Verification items for the finished model (mm, model axes). Face numbers are marked on the shaded views. Round coordinates to 2 decimals unless told otherwise and drop trailing zeros. Loops run counter-clockwise (first coordinate to the right, second up) from the corner with the lowest first, then second, coordinate; pieces in that order, holes last. Notation, with made-up numbers: M 68,-32.5 L 119,-32.5 A30 cw 119,5.5 Z; hole C -5.5,-2.75 d1. An arc over 180 degrees is marked long. One line per item, written item: value.
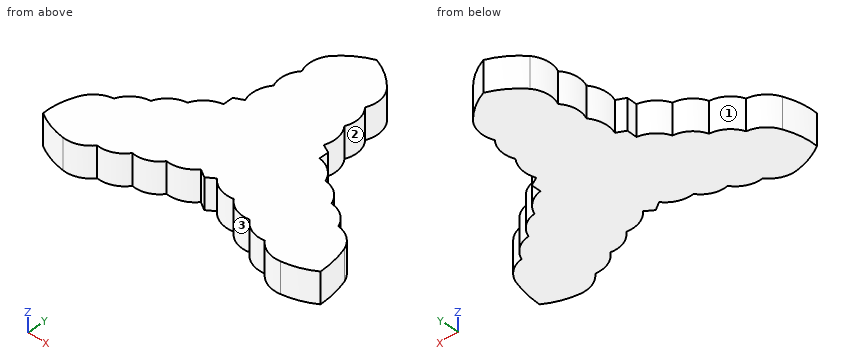
from build123d import *

# Parameters (mm, degrees)
F1_DEPTH = 7.9375


# Not quite as in the source:
# - a length typed as a fraction of an inch, garbled in the dataset ("3 / 203.2 mm" for 3/8 in), is restored


with BuildPart() as f1:
    # F0 (on Top) → F1 (new body)
    with BuildSketch(Plane.XY):
        with BuildLine():
            ThreePointArc((-0.0986067535, 34.0497419238), (-4.0682176485, 31.9659465467), (-7.4162920937, 28.9842672646))
            ThreePointArc((-7.4162920937, 28.9842672646), (-8.8119305122, 25.5953281623), (-8.2258973271, 21.977417171))
            ThreePointArc((-8.2258973271, 21.977417171), (-9.7181261566, 18.698842434), (-9.2097157612, 15.1327075437))
            ThreePointArc((-9.2097157612, 15.1327075437), (-10.6205392688, 11.8246856933), (-10.2093555033, 8.2519613206))
            Line((-10.2093555033, 8.2519613206), (-12.369341217, 7.1464567445))
            Line((-12.369341217, 7.1464567445), (-12.369341217, 4.6386048198))
            Line((-12.369341217, 4.6386048198), (-12.369341217, 4.5682978211))
            ThreePointArc((-12.369341217, 4.5682978211), (-15.5930977879, 3.1185654947), (-17.7027139134, 0.2823972963))
            ThreePointArc((-17.7027139134, 0.2823972963), (-21.0452825194, -1.0603738309), (-23.1384971151, -3.9919692741))
            ThreePointArc((-23.1384971151, -3.9919692741), (-26.5647165348, -5.2934051439), (-28.80180468, -8.19653302))
            ThreePointArc((-28.80180468, -8.19653302), (-32.1117440701, -9.5846599904), (-34.254974256, -12.4637500588))
            ThreePointArc((-34.254974256, -12.4637500588), (-35.4454588739, -16.4293701566), (-35.6585793197, -20.564340055))
            ThreePointArc((-35.6585793197, -20.564340055), (-31.9389059128, -22.4150036937), (-27.9142765499, -23.4461606411))
            ThreePointArc((-27.9142765499, -23.4461606411), (-24.3492963179, -23.0296138883), (-21.4921734029, -20.8571857766))
            ThreePointArc((-21.4921734029, -20.8571857766), (-17.8594468391, -20.3713745504), (-15.0192606046, -18.054899429))
            ThreePointArc((-15.0192606046, -18.054899429), (-11.4338171794, -17.7079201351), (-8.5996589687, -15.484556372))
            ThreePointArc((-8.5996589687, -15.484556372), (-5.0294162563, -15.0523544446), (-2.1409380715, -12.9098966718))
            Line((-2.1409380715, -12.9098966718), (0, -14.2561570176))
            Line((0, -14.2561570176), (1.9696742658, -12.9098966718))
            ThreePointArc((1.9696742658, -12.9098966718), (4.9392756736, -15.0084468105), (8.560301624, -15.3410370587))
            ThreePointArc((8.560301624, -15.3410370587), (11.3944598347, -17.5644008218), (14.9799032599, -17.9113801157))
            ThreePointArc((14.9799032599, -17.9113801157), (17.8200894944, -20.2278552371), (21.4528160582, -20.7136664634))
            ThreePointArc((21.4528160582, -20.7136664634), (24.3099389732, -22.886094575), (27.8749192052, -23.3026413279))
            ThreePointArc((27.8749192052, -23.3026413279), (31.8832272801, -22.3269581873), (35.5659238994, -20.4678624868))
            ThreePointArc((35.5659238994, -20.4678624868), (35.2059818343, -16.3418066269), (34.2156169113, -12.3202307456))
            ThreePointArc((34.2156169113, -12.3202307456), (32.0723867254, -9.4411406771), (28.7624473353, -8.0530137067))
            ThreePointArc((28.7624473353, -8.0530137067), (26.5253591901, -5.1498858306), (23.0991397704, -3.8484499608))
            ThreePointArc((23.0991397704, -3.8484499608), (21.0059251747, -0.9168545176), (17.6633565687, 0.4259166096))
            ThreePointArc((17.6633565687, 0.4259166096), (15.4847616458, 3.3168082822), (12.1560195839, 4.739132713))
            Line((12.1560195839, 4.739132713), (12.1560195839, 7.1464567445))
            Line((12.1560195839, 7.1464567445), (9.9960338703, 8.2519613206))
            ThreePointArc((9.9960338703, 8.2519613206), (10.4072176357, 11.8246856933), (8.9963941282, 15.1327075437))
            ThreePointArc((8.9963941282, 15.1327075437), (9.5048045235, 18.698842434), (8.012575694, 21.977417171))
            ThreePointArc((8.012575694, 21.977417171), (8.5986088792, 25.5953281623), (7.2029704606, 28.9842672646))
            ThreePointArc((7.2029704606, 28.9842672646), (3.8655773676, 31.9687453881), (-0.0986067535, 34.0497419238))
        make_face()
    extrude(amount=F1_DEPTH)


solid = f1.part
(1) Sectioned sample at B-B on y = 19.5. Enter the section's corners in (x, z), and give its area (3 significant figures).
Completed:
outline: M -9.55,0 L 9.34,0 L 9.34,7.94 L -9.55,7.94 Z
area: 150 mm^2
(2) Thickness scan on L1, parallel to X at y = -13.5, z = 5; L2, parallel to X at y = -16, z = 3.75; L3, parallel to Y at x = 27, z = 3.25. Record the ranges inside material, lowest first. Write a range as from..to.
Completed:
L1: x = -34.67..-2.67, -1.2..1.11, 2.52..34.58
L2: x = -35.37..-9.01, 9.1..35.15
L3: y = -23.38..-5.54
(3) Sectioned sample at C-C on x = 24.5. Enter the section's corners in (y, z), and give its area (3 significant figures).
Completed:
outline: M -22.96,0 L -4.12,0 L -4.12,7.94 L -22.96,7.94 Z
area: 150 mm^2
(4) Depth check by flat-ended pin: pin 1 Ø2 at (y, z) = (6.5, 5.5) entering from -X; pin 2 Ø3 at (y, z) = (2, 1.5) entering from +X; pin 3 Ø3 at (y, z) = (-9, 1) entering from -X. Enter the tip coordinate at first touch or a pass-through.
Completed:
pin 1: stops at x = -12.37
pin 2: stops at x = 17.63
pin 3: stops at x = -33.07
(5) Mould release check, pull along Y, two halves, no side actions. Record for the marked faces 1, 2 and 3: +Y half, -Y half, draft (parallel to the pull), parting line (faces both ways), or undercut.
Completed:
face 1: +Y half
face 2: undercut
face 3: -Y half
